Here's how the part is built. I have some questions about the finished solid (model axes, mm). Face numbers are marked on the shaded views. Round coordinates to 2 decimals unless told otherwise and drop trailing zeros. Order: outer loops, then holes, each group sorted by start corner. A loop starts at its lowest first (then second) coordinate and runs counter-clockwise, first axis right, second up. Notation, with made-up numbers: (-35.75, 27) -> (-30.75, 27) arc R18 ccw to (-30.75, 46) -> close; hole circle Ø9 at (43, 29). An arc over 180 degrees is marked (long way). One line per item, written item: value.
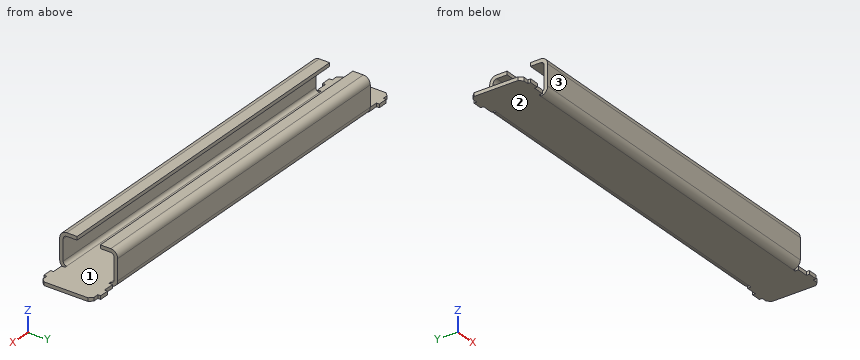
```python
from build123d import *

# Parameters (mm, degrees)
BOSS_EXTRUDE1_DEPTH = 150
FILLET1_R           = 6
FILLET2_R           = 3
BOSS_EXTRUDE2_DEPTH = 3


with BuildPart() as part:
    # Sketch2 → Boss-Extrude1 (new body, symmetric)
    with BuildSketch(Plane(origin=(0, 0, 0), x_dir=(0, 0, -1), z_dir=(1, 0, 0))):
        Polygon((0, 0), (30, 0), (30, 50), (0, 50), (0, 35), (3, 35), (3, 47), (27, 47), (27, 3), (3, 3), (3, 15), (0, 15), align=None)
    extrude(amount=BOSS_EXTRUDE1_DEPTH, both=True)

    # Fillet1
    fillet1_edges = [part.edges().sort_by_distance(p)[0] for p in [
        (0, 50, 0),
        (0, 50, -30),
        (0, 0, -30),
        (0, 0, 0),
    ]]
    fillet(fillet1_edges, radius=FILLET1_R)

    # Fillet2
    fillet2_edges = [part.edges().sort_by_distance(p)[0] for p in [
        (0, 3, -3),
        (0, 3, -27),
        (0, 47, -27),
        (0, 47, -3),
    ]]
    fillet(fillet2_edges, radius=FILLET2_R)

    # Sketch3 → Boss-Extrude2 (add)
    with BuildSketch(Plane.XY.offset(-27)):
        Polygon((-150, 44), (-152, 44), (-152, 47), (-161.5, 47), (-161.5, 49.5), (-169.5, 49.5), (-169.5, 47), (-174, 47), (-177, 44), (-177, 6), (-174, 3), (-169.5, 3), (-169.5, 0.5), (-161.5, 0.5), (-161.5, 3), (-152, 3), (-152, 6), (-150, 6), align=None)
        Polygon((174, 3), (177, 6), (177, 44), (174, 47), (169.5, 47), (169.5, 49.5), (161.5, 49.5), (161.5, 47), (152, 47), (152, 44), (150, 44), (150, 6), (152, 6), (152, 3), (161.5, 3), (161.5, 0.5), (169.5, 0.5), (169.5, 3), align=None)
    extrude(amount=-BOSS_EXTRUDE2_DEPTH)


solid = part.part
```
Q1. I want a section at C-C on y = 25. Write out the boundary of the cut face in (x, z).
Answers:
outline: (-177, -30) -> (177, -30) -> (177, -27) -> (-177, -27) -> close
Q2. I want a section at D-D on x = 155.5. Write out the boundary of the cut face in (y, z).
Answers:
outline: (3, -30) -> (47, -30) -> (47, -27) -> (3, -27) -> close
Q3. For P1, Ø3.5, axis at x = 171.5, z = -29, coming from the -Y side; P2, Ø0.9, axis at x = 166, z = -28.5, coming from the -Y side; P3, Ø1.5, axis at x = -172, z = -28.5, coming from the +Y side, each with a flat end and sliding along its axis, tell me the tip position at first contact or that it passes through.
Answers:
P1: y = 3
P2: y = 0.5
P3: y = 47
Q4. I need wall thicknesses on line 1 along Z through (x, y) = (-76, 10.5); line 2 along Y through (x, z) = (11, -11.5); line 3 along Z through (x, y) = (153, 39). Which ranges of each line are inside material? Lowest first, please.
Answers:
line 1: -30 to -27, -3 to 0
line 2: 0 to 3, 47 to 50
line 3: -30 to -27
Q5. If we mould it in two halves opening along Y, with no side actions, what happens to the marked faces 1, 2 and 3? For each: pulls with the +Y half, pulls with the -Y half, needs draft (parallel to the pull), parting line crosses it, or undercut.
Answers:
face 1: undercut
face 2: needs draft
face 3: pulls with the -Y half
Q6. I want a section at A-A on z = -12.75. Write out the boundary of the cut face in (x, y).
Answers:
outline: (-150, 0) -> (150, 0) -> (150, 3) -> (-150, 3) -> close; (-150, 47) -> (150, 47) -> (150, 50) -> (-150, 50) -> close
Q7. I want a section at B-B on x = -47. Write out the boundary of the cut face in (y, z).
Answers:
outline: (0, -24) arc R6 ccw to (6, -30) -> (44, -30) arc R6 ccw to (50, -24) -> (50, -6) arc R6 ccw to (44, 0) -> (35, 0) -> (35, -3) -> (44, -3) arc R3 cw to (47, -6) -> (47, -24) arc R3 cw to (44, -27) -> (6, -27) arc R3 cw to (3, -24) -> (3, -6) arc R3 cw to (6, -3) -> (15, -3) -> (15, 0) -> (6, 0) arc R6 ccw to (0, -6) -> close
